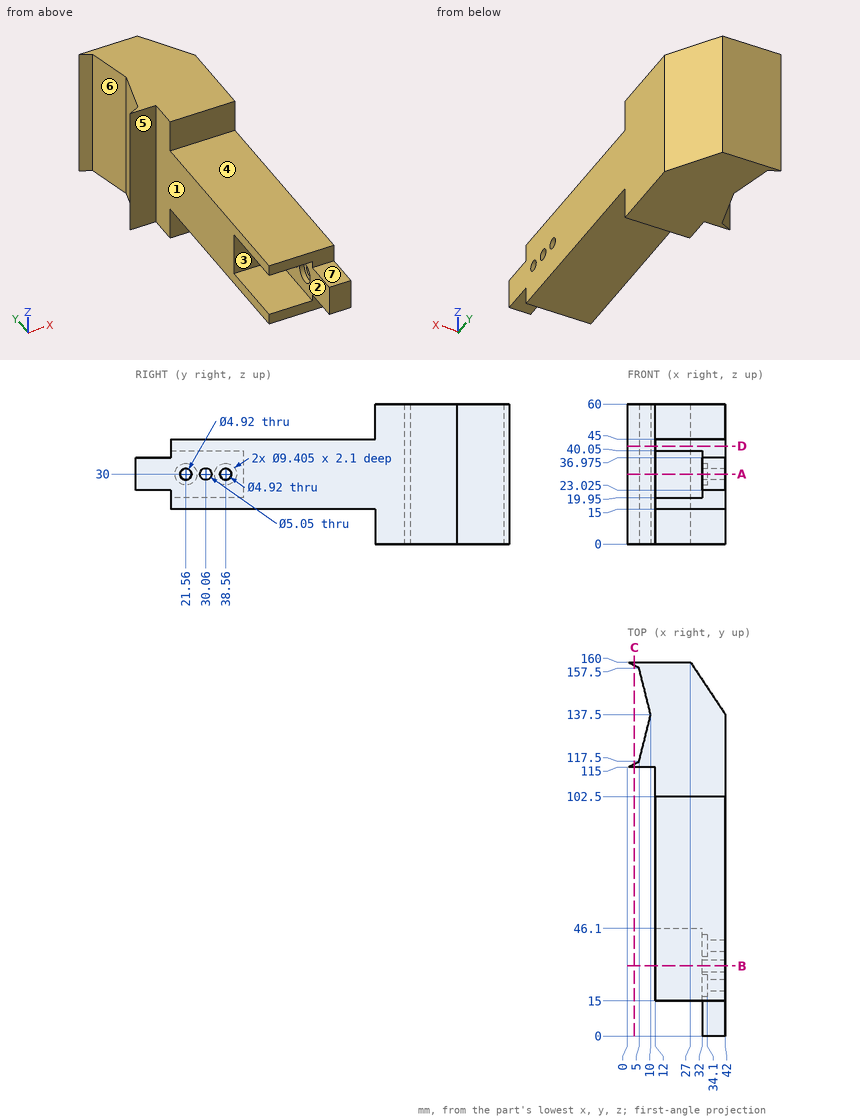
Design review of the part shown in the three views and the two pictorial views. Dimensions are in mm from the part's minimum x, y and z. A direction names the side the tool comes from. Give positions to 0.01 mm unless a question says otherwise; leave off trailing zeros. Order: outer loops, then holes, each group sorted by start corner. A loop starts at its lowest first (then second) coordinate and runs counter-clockwise, first axis right, second up. Notation, with made-up numbers: M -34.75,63.25 L 14.25,63.25 A9 ccw 14.25,80.25 Z; hole C -7.75,28.5 d11. An arc over 180 degrees is marked long. Answer in a Markdown table with one row per item. Add a question column.
(1) Consider section B-B on y = 30.06. State the section outline as (x, z) points (3 decimals), and give its area (4 significant figures).
(2) Mouldability with a two-part tool opening along Z and no side actions: class the marked faces 1, 2, 3 and 4 as +Z half, -Z half, draft (parallel to the pull), parting line (faces both ways), or undercut.
(3) Wall thickness on probe 1 along Y at (x, z) = (40.5, 30) (3 decimals); probe 2 along Z at (x, y) = (22.5, 35.5); probe 3 along Y at (x, z) = (38.5, 30) (3 decimals): over which ranges is each line inside the solid? List them lowest first. Write a range as [from, to].
(4) Consider section A-A on z = 30. Give the number of separate pieces and of enclosed holes in the cut face, and give its area (3 significant figures).
(5) Consider section C-C on x = 3. State the section outline as (y, z) points.
(6) Consider section D-D on z = 42. State the section outline as (x, y) points, and give its area (3 significant figures).
(7) For the marked faces 5, 6 and 7, list the 3-axis set-ups (+Z, -Z, +X, -X, +Y, -Y) from which the entire face can be reached by the end or side of a thin tool; tool diameter is ignored.
(8) For pin 1 (6 mm diameter, centred on y = 53.5, z = 10.5, fed in from -X); pin 2 (24 mm diameter, centred on x = 20, y = 79.5, fed in from -Z); pin 3 (16 mm diameter, centred on y = 15.5, z = 30, fed in from -X); pin 4 (1 mm diameter, centred on y = 99.5, z = 28.5, fed in from -X), all flat-tipped, find the tip position at first contact; note any pin that passes through.
Evaluation:
| question | item | result |
|---|---|---|
| 1 | outline | M 12,15 L 42,15 L 42,27.475 L 32,27.475 L 32,19.95 L 12,19.95 Z; M 12,40.05 L 32,40.05 L 32,32.525 L 42,32.525 L 42,45 L 12,45 Z |
| 1 | area | 447.5 mm^2 |
| 2 | face 1 | draft |
| 2 | face 2 | undercut |
| 2 | face 3 | undercut |
| 2 | face 4 | +Z half |
| 3 | probe 1 | y = [0, 19.1], [24.02, 27.535], [32.585, 36.1], [41.02, 139.75] |
| 3 | probe 2 | z = [15, 19.95], [40.05, 45] |
| 3 | probe 3 | y = [0, 19.1], [24.02, 27.535], [32.585, 36.1], [41.02, 142.75] |
| 4 | separate pieces | 4 |
| 4 | enclosed holes | 0 |
| 4 | area | 3,770 mm^2 |
| 5 | outline | M 115,0 L 116.5,0 L 116.5,60 L 115,60 Z; M 158.5,0 L 160,0 L 160,60 L 158.5,60 Z |
| 6 | outline | M 0,115 L 12,115 L 12,15 L 42,15 L 42,137.5 L 27,160 L 0,160 L 5,157.5 L 10,137.5 L 5,117.5 Z |
| 6 | area | 4,410 mm^2 |
| 7 | face 5 | +Z, -Z, -X, -Y |
| 7 | face 6 | +Z, -Z, -X |
| 7 | face 7 | +Z, +X, -X, -Y |
| 8 | pin 1 | passes through |
| 8 | pin 2 | stops at z = 15 |
| 8 | pin 3 | stops at x = 32 |
| 8 | pin 4 | stops at x = 12 |
